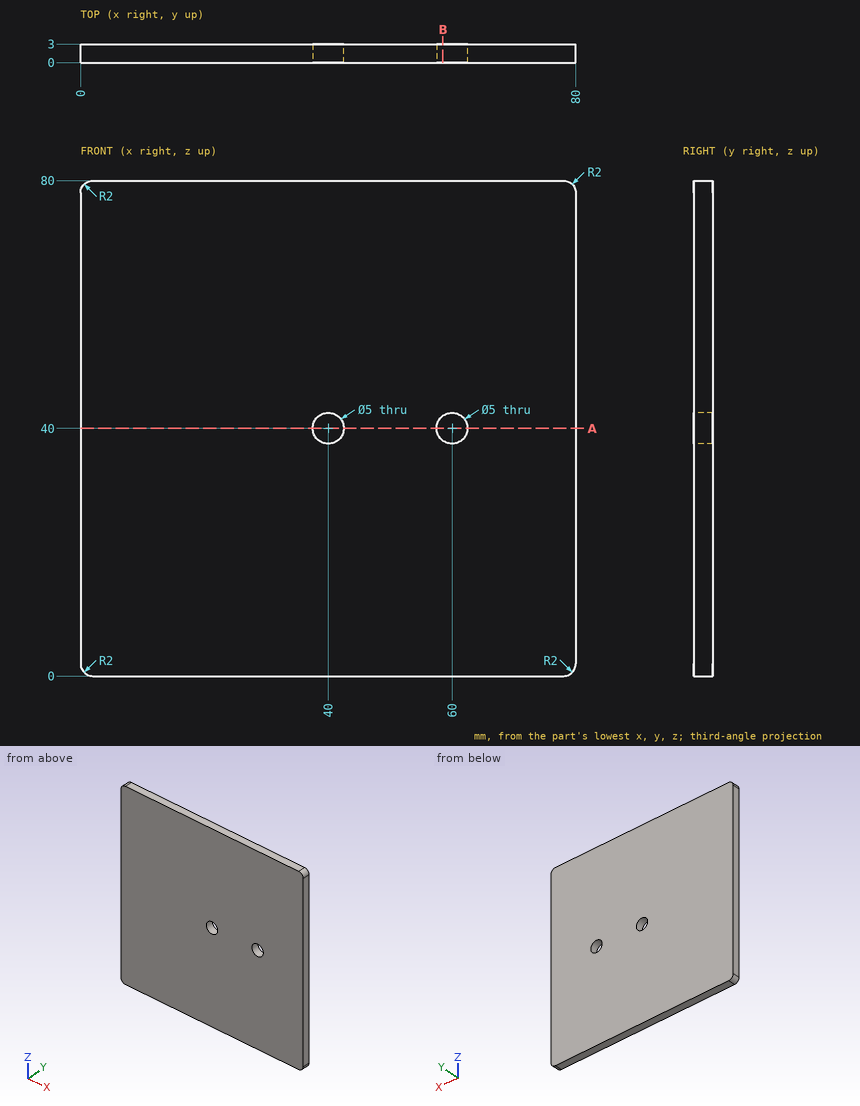
Here's the drawing with two shaded views (mm, measured from the low corner). I have some questions. Give positions to 0.01 mm unless a question says otherwise; leave off trailing zeros. Order: outer loops, then holes, each group sorted by start corner. A loop starts at its lowest first (then second) coordinate and runs counter-clockwise, first axis right, second up. Notation, with made-up numbers: (-23.75, 41.5) -> (14.25, 41.5) arc R14 ccw to (14.25, 49.5) -> close; hole circle Ø6 at (59.5, -8.75). An arc over 180 degrees is marked (long way). Use a Markdown table: item, result. Add a question column.
Item 1: Imagine slicing it at A-A on z = 40. Please give me the cut outline in (x, y), plus the area to 3 significant figures.
Item 2: I need wall thicknesses on line 1 (X direction, y = 1.75, z = 40); line 2 (Z direction, x = 60, y = 1.8); line 3 (X direction, y = 1.95, z = 42). Which ranges of each line are inside material? Lowest first, please.
Item 3: Imagine slicing it at B-B on x = 58.5. Please give me the cut outline in (y, z).
Item 4: Will this pin go through, and if not, where does the flat tip stop? pin 1 (4 mm diameter, centred on x = 60, z = 40, fed in from -Y).
Data:
| question | item | result |
|---|---|---|
| 1 | outline | (0, 0) -> (37.5, 0) -> (37.5, 3) -> (0, 3) -> close; (42.5, 0) -> (57.5, 0) -> (57.5, 3) -> (42.5, 3) -> close; (62.5, 0) -> (80, 0) -> (80, 3) -> (62.5, 3) -> close |
| 1 | area | 210 mm² |
| 2 | line 1 | x = 0 to 37.5, 42.5 to 57.5, 62.5 to 80 |
| 2 | line 2 | z = 0 to 37.5, 42.5 to 80 |
| 2 | line 3 | x = 0 to 38.5, 41.5 to 58.5, 61.5 to 80 |
| 3 | outline | (0, 0) -> (3, 0) -> (3, 38) -> (0, 38) -> close; (0, 42) -> (3, 42) -> (3, 80) -> (0, 80) -> close |
| 4 | pin 1 | passes through |
